Can you work these out from the model? Positions are in its coordinate system, mm. Coordinates: 2 decimals unless noted, no trailing zeros. Write each loop counter-clockwise with the first axis right and the second up, starting at its lowest first coordinate (ties: lowest second). Pieces come first, ordered by that corner, then holes. Notation, with made-up numbers: (34.25, -1) - (78.25, -1) arc R13 ccw to (78.25, 18) - close; hole circle Ø4 at (85.5, 84). An arc over 180 degrees is marked (long way). Use one line per item in the form item = value. Start each with the question number.
(1) For pin 1 Ø1.5 at (x, y) = (536.5, 1.5) entering from -Z, with a flat end and sliding along its axis, tell me the tip position at first contact or that it passes through.
(2) If we section it at A-A on y = 0.8: Please give me the cut outline in (x, z).
(3) If we section it at B-B on x = 5.5: Please give me the cut outline in (y, z), then the cut area to 3 significant figures.
(4) If I drill on probe 1 along Z at (x, y) = (337, 0.4), over which ranges is the centre line in solid material (lowest first)? Write a range as from..to.
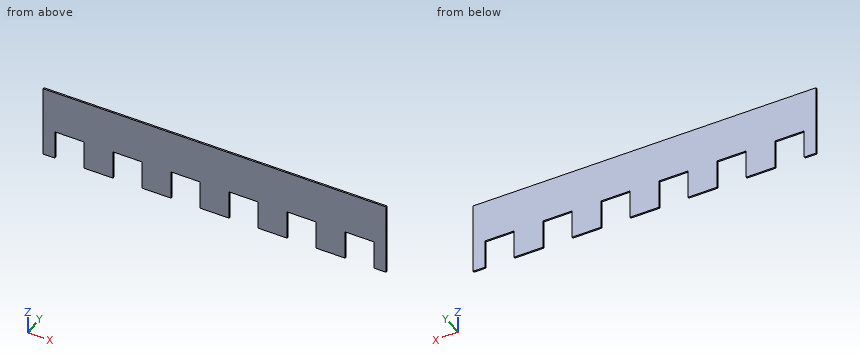
```python
from build123d import *

# Parameters (mm, degrees)
SKETCH1_W               = 650
SKETCH1_H               = 137
BOSS_EXTRUDE1_DEPTH     = 3
CUT_EXTRUDE2_DEPTH      = 598.701122593
CUT_EXTRUDE2_DEPTH_BACK = 598.701122593
SKETCH2_W               = 55
SKETCH2_H               = 55
SKETCH3_W               = 55
SKETCH3_H               = 55
CUT_EXTRUDE3_DEPTH      = 598.701122593


with BuildPart() as part:
    # Sketch1 → Boss-Extrude1 (new body)
    with BuildSketch(Plane(origin=(0, 0, 0), x_dir=(1, 0, 0), z_dir=(0, 1, 0))):
        with Locations((262.487315064, 41.483119558)):
            Rectangle(SKETCH1_W, SKETCH1_H)
    extrude(amount=BOSS_EXTRUDE1_DEPTH)

    # Sketch2 → Cut-Extrude2 (cut, two sides: drawn at the far end of the back side and taken through both)
    with BuildSketch(Plane(origin=(0, 0, 0), x_dir=(1, 0, 0), z_dir=(0, 1, 0)).offset(-CUT_EXTRUDE2_DEPTH_BACK)):
        with Locations((97.487315064, 82.483119558)):
            Rectangle(SKETCH2_W, SKETCH2_H)
        with Locations((207.487315064, 82.483119558)):
            Rectangle(SKETCH2_W, SKETCH2_H)
        with Locations((317.487315064, 82.483119558)):
            Rectangle(SKETCH2_W, SKETCH2_H)
        with Locations((427.487315064, 82.483119558)):
            Rectangle(SKETCH2_W, SKETCH2_H)
        with Locations((537.487315064, 82.483119558)):
            Rectangle(SKETCH2_W, SKETCH2_H)
    extrude(amount=CUT_EXTRUDE2_DEPTH + CUT_EXTRUDE2_DEPTH_BACK, mode=Mode.SUBTRACT)

    # Sketch3 → Cut-Extrude3 (cut, through all)
    with BuildSketch(Plane(origin=(0, 3, 0), x_dir=(1, 0, 0), z_dir=(0, 1, 0))):
        with Locations((-12.512684936, 82.483119558)):
            Rectangle(SKETCH3_W, SKETCH3_H)
    extrude(amount=-CUT_EXTRUDE3_DEPTH, mode=Mode.SUBTRACT)


solid = part.part
```
Reported:
q1.pin_1 = -54.98
q2.outline = (-62.51, -109.98) - (-40.01, -109.98) - (-40.01, -54.98) - (14.99, -54.98) - (14.99, -109.98) - (69.99, -109.98) - (69.99, -54.98) - (124.99, -54.98) - (124.99, -109.98) - (179.99, -109.98) - (179.99, -54.98) - (234.99, -54.98) - (234.99, -109.98) - (289.99, -109.98) - (289.99, -54.98) - (344.99, -54.98) - (344.99, -109.98) - (399.99, -109.98) - (399.99, -54.98) - (454.99, -54.98) - (454.99, -109.98) - (509.99, -109.98) - (509.99, -54.98) - (564.99, -54.98) - (564.99, -109.98) - (587.49, -109.98) - (587.49, 27.02) - (-62.51, 27.02) - close
q3.outline = (0, -54.98) - (3, -54.98) - (3, 27.02) - (0, 27.02) - close
q3.area = 246 mm2
q4.probe_1 = -54.98..27.02
